Design review of the part built by this model. Coordinates are the model's own, in mm. Coordinates: 2 decimals unless noted, no trailing zeros. Loops run counter-clockwise (first coordinate to the right, second up) from the corner with the lowest first, then second, coordinate; pieces in that order, holes last. Notation, with made-up numbers: (30.25, 81) -> (58.25, 81) arc R37 ccw to (58.25, 117) -> close; hole circle Ø4 at (5.5, 70). An arc over 180 degrees is marked (long way). Use a Markdown table: item, result. Add a question column.
Q1. Take a section at A-A on y = -784. Write out the cut boundary in (x, z).
Q2. For probe 1 along Y at (x, z) = (1.25, 532); probe 2 along Y at (x, z) = (15, 410), list the stretches that pass through material, from the lowest coordinate up.
Q3. Take a section at C-C on z = 622. Write out the cut boundary in (x, y).
Q4. Take a section at B-B on x = 9.5. Write out the cut boundary in (y, z) (1 decimal), plus the area to 3 significant figures.
Q5. Clearance check with flat-ended pins moving along their axes: pin 1 Ø8.5 at (y, z) = (-784.46, 698.96) entering from -X; pin 2 Ø1.5 at (x, z) = (15, 481.5) entering from +Y; pin 3 Ø1 at (x, y) = (10.5, -759) entering from -Z; pin 4 Ø2 at (x, z) = (11, 502.5) entering from +Y. State where each tip first meets the part, or that it passes through.
Q6. Draft analysis for pull direction Y (two halves, no side actions). For faces 1 (the face through (9.392, -745.204, 257.251)), 2 (the face through (9.39, -749.03, 243.14)), 3 (the face through (9.4, -754.2, 475.3)), state which applies: pulls with the +Y half, pulls with the -Y half, needs draft (parallel to the pull), parting line crosses it, or undercut.
from build123d import *

# Parameters (mm, degrees)
F2_R     = 4.7625
F3_DEPTH = 19.05


with BuildPart() as f3:
    # F2 (on Right) → F3 (new body)
    with BuildSketch(Plane.YZ):
        with BuildLine():
            ThreePointArc((-771.797877, 699.955234), (-785.45089, 711.62465), (-797.120305, 697.971637))
            Line((-797.120305, 697.971637), (-762.407361, 254.829153))
            ThreePointArc((-762.407361, 254.829153), (-748.754349, 243.159737), (-737.084934, 256.81275))
            Line((-737.084934, 256.81275), (-771.797877, 699.955234))
        make_face()
        with Locations((-749.746147, 255.820951)):
            Circle(F2_R, mode=Mode.SUBTRACT)
        with Locations((-784.459091, 698.963436)):
            Circle(F2_R, mode=Mode.SUBTRACT)
    extrude(amount=F3_DEPTH)


solid = f3.part
Answer list:
| question | item | result |
|---|---|---|
| 1 | outline | (0, 530.48) -> (19.05, 530.48) -> (19.05, 694.22) -> (0, 694.22) -> close; (0, 703.7) -> (19.05, 703.7) -> (19.05, 711.66) -> (0, 711.66) -> close |
| 2 | probe 1 | -784.12 to -758.64 |
| 2 | probe 2 | -774.56 to -749.08 |
| 3 | outline | (0, -791.17) -> (19.05, -791.17) -> (19.05, -765.69) -> (0, -765.69) -> close |
| 4 | outline | (-797.1, 698) -> (-762.4, 254.8) arc R12.7 ccw to (-737.1, 256.8) -> (-771.8, 700) arc R12.7 ccw to start; hole circle Ø9.5 at (-784.5, 699); hole circle Ø9.5 at (-749.7, 255.8) |
| 4 | area | 11,700 mm² |
| 5 | pin 1 | through |
| 5 | pin 2 | y = -754.63 |
| 5 | pin 3 | z = 246.62 |
| 5 | pin 4 | y = -756.25 |
| 6 | face 1 | undercut |
| 6 | face 2 | parting line crosses it |
| 6 | face 3 | pulls with the +Y half |
